Here's the drawing with two shaded views (mm, measured from the low corner). I have some questions. Coordinates: 2 decimals unless noted, no trailing zeros. Loops run counter-clockwise (first coordinate to the right, second up) from the corner with the lowest first, then second, coordinate; pieces in that order, holes last. Notation, with made-up numbers: (87, 13) - (112, 13) arc R31 ccw to (112, 50) - close; hole circle Ø6 at (75, 46). An arc over 180 degrees is marked (long way). One line per item, written item: value. Start each with the question number.
(1) If I drill on line 1 along X through (y, z) = (2.35, 8); line 2 along X through (y, z) = (1.95, 25); line 3 along Z through (x, y) = (10, 1.1), over which ranges is the centre line in solid material (lowest first)? Write a range as from..to.
(2) If we section it at B-B on z = 25: Write out the boundary of the cut face in (x, y), then the cut area to 3 significant figures.
(3) If we section it at C-C on y = 0.85: Write out the boundary of the cut face in (x, z).
(4) If we section it at A-A on x = 27: Write out the boundary of the cut face in (y, z), then the cut area to 3 significant figures.
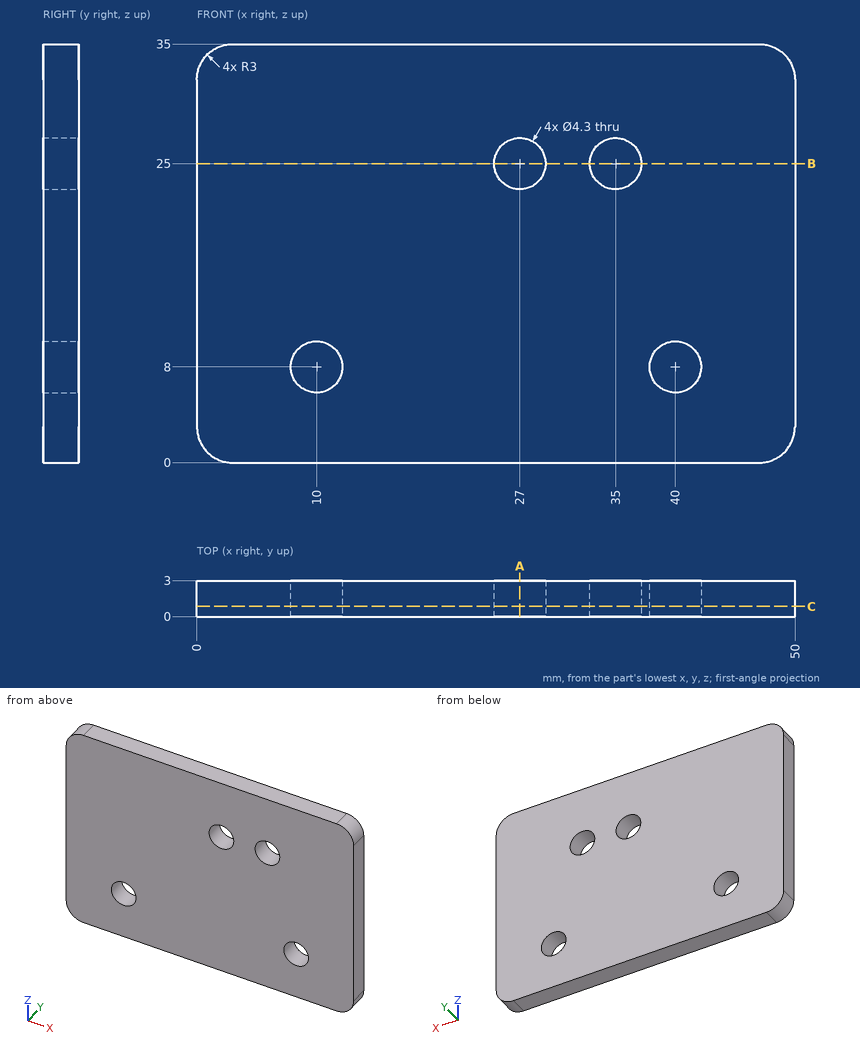
Values:
1. line 1: x = 0..7.85, 12.15..37.85, 42.15..50
1. line 2: x = 0..24.85, 29.15..32.85, 37.15..50
1. line 3: z = 0..5.85, 10.15..35
2. outline: (0, 0) - (24.85, 0) - (24.85, 3) - (0, 3) - close; (29.15, 0) - (32.85, 0) - (32.85, 3) - (29.15, 3) - close; (37.15, 0) - (50, 0) - (50, 3) - (37.15, 3) - close
2. area: 124 mm2
3. outline: (0, 3) arc R3 ccw to (3, 0) - (47, 0) arc R3 ccw to (50, 3) - (50, 32) arc R3 ccw to (47, 35) - (3, 35) arc R3 ccw to (0, 32) - close; hole circle Ø4.3 at (10, 8); hole circle Ø4.3 at (27, 25); hole circle Ø4.3 at (35, 25); hole circle Ø4.3 at (40, 8)
4. outline: (0, 0) - (3, 0) - (3, 22.85) - (0, 22.85) - close; (0, 27.15) - (3, 27.15) - (3, 35) - (0, 35) - close
4. area: 92.1 mm2
